Read the model definition and answer for the solid it produces. Units are mm, in the model's axes. Coordinates: 2 decimals unless noted, no trailing zeros. Write each loop counter-clockwise with the first axis right and the second up, starting at its lowest first coordinate (ties: lowest second). Pieces come first, ordered by that corner, then holes.
1) The part is cut by section A-A (x = 23.5). Determine the outline of the cut face in (y, z), then the cut area to 3 significant figures.
2) Each of these flat-tipped pins is pushed along its axis until it touches: pin 1 Ø1 at (x, y) = (-4, -1) entering from +Z; pin 2 Ø2 at (x, y) = (-21, -0.5) entering from -Z. Where does it stop, or does it pass through?
3) Find the intervals of material crossed by line 1 (X direction, y = -0.5, z = -0.4); line 2 (Z direction, x = 2.5, y = -0.05); line 3 (Y direction, x = 14, z = 0.2), in increasing order.
Autodesk Inventor part; units mm, degrees
ref_plane "YZ Plane" through (0, 0, 0) normal (1, 0, 0) x (0, 1, 0)
ref_plane "XZ Plane" through (0, 0, 0) normal (0, 1, 0) x (-1, 0, 0)
ref_plane "XY Plane" through (0, 0, 0) normal (0, 0, 1) x (1, 0, 0)
sketch "Sketch1" plane through (0, 0, 0) normal (1, 0, 0) x (0, 1, 0)
  circle A0 centre (0, 0) radius 2
  circle A1 centre (0, 0) radius 2.2361
  dimension "d0" = 4
extrude "Extrusion1" add sketch "Sketch1" along normal mid plane 63 contours A0
sketch "Sketch2" plane through (31.5, 0, 0) normal (1, 0, 0) x (0, 0, -1)
  circle A0 centre (0, 0) radius 2.3871
extrude "Extrusion2" add sketch "Sketch2" against normal blind 1.5
fillet "Fillet1" radius 2 1 edges at (31.5, 0, 2.3871)
mirror "Mirror1" about plane through (0, 0, 0) normal (1, 0, 0) of "Extrusion2", "Fillet1"
ref_plane "Work Plane1" through (0, 0, 0) normal (1, 0, 0) x (0, 1, 0)
properties part number "clampScrewHandle" material "Steel, Alloy"
Reported:
1. outline: circle Ø4 at (0, 0)
1. area: 12.6 mm2
2. pin 1: stops at z = 1.94
2. pin 2: stops at z = -2
3. line 1: x = -31.49 to 31.49
3. line 2: z = -2 to 2
3. line 3: y = -1.99 to 1.99
